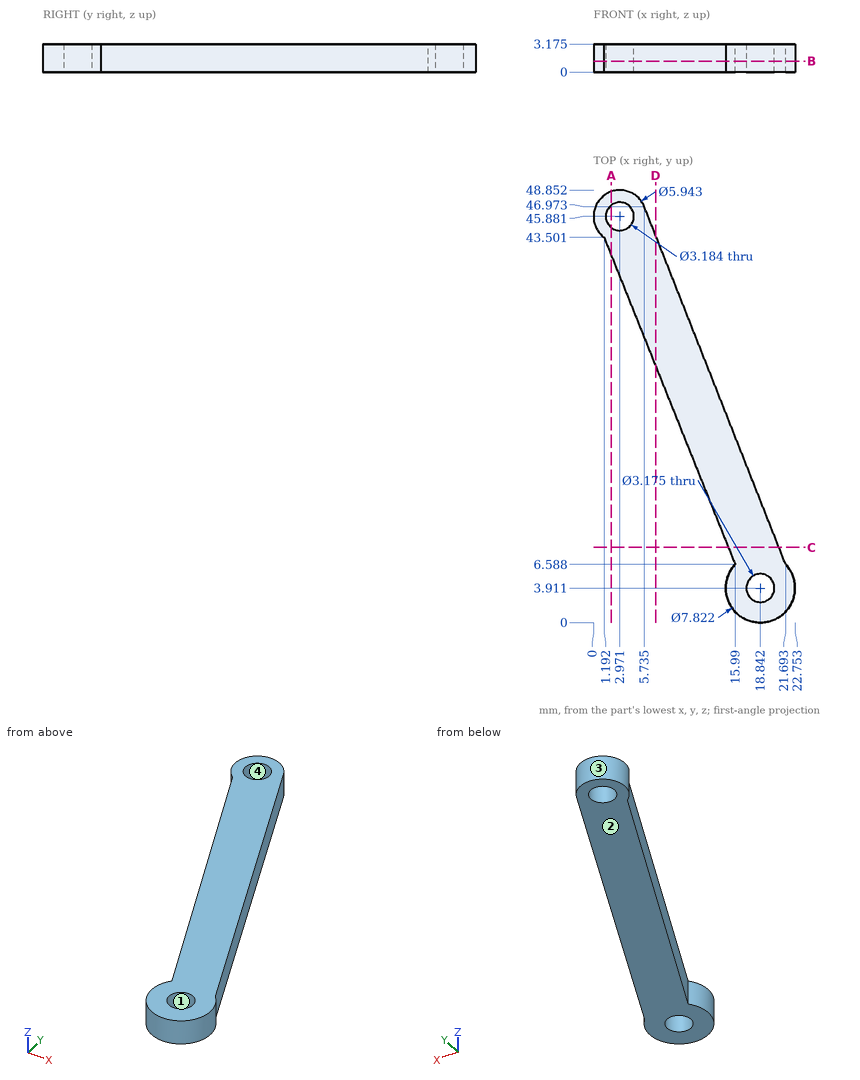
Print and shaded views of the part. All mm, measured from the part's lowest x, y and z. Coordinates: 2 decimals unless noted, no trailing zeros. Loops run counter-clockwise (first coordinate to the right, second up) from the corner with the lowest first, then second, coordinate; pieces in that order, holes last. Notation, with made-up numbers: (75.5, 61) - (121.5, 61) arc R22 ccw to (121.5, 88) - close; hole circle Ø6 at (85, 26). An arc over 180 degrees is marked (long way). Use one line per item in the form item = value. Start each with the question number.
1) Two-plate mould, pull along Y, no slides. Class the marked faces 1, 2, 3 and 4: +Y half, -Y half, draft (parallel to the pull), parting line (faces both ways), or undercut.
2) Band-saw the part on A-A (x = 2). Give the cut face in (y, z) (1 decimal).
3) Drill centre lines: L1, parallel to Y at x = 1.75, z = 2.7 (1 decimal); L2, parallel to X at y = 28.5, z = 0.15 (1 decimal); L3, parallel to X at y = 12.5, z = 3. Where is each one in solid material? Low to high. Write a range as from..to.
4) Band-saw the part on C-C (y = 8.5). Give the cut face in (x, z) (1 decimal).
5) Flat gauge pins, fed straight in: pin 1 (1 mm diameter, centred on x = 17, z = 2.5, fed in from -Y); pin 2 (2.5 mm diameter, centred on x = 2.97, y = 45.88, fed in from -Z). Where does each tip first touch, or does it go through?
6) Band-saw the part on D-D (x = 7). Give the cut face in (y, z) (1 decimal).
7) Band-saw the part on B-B (z = 1.25). Give the cut face in (x, y) (1 decimal), and give its area (3 significant figures).
Check values:
q1.face_1 = undercut
q1.face_2 = draft
q1.face_3 = parting line
q1.face_4 = undercut
q2.outline = (41.5, 0) - (44.6, 0) - (44.6, 3.2) - (41.5, 3.2) - close; (47.1, 0) - (48.7, 0) - (48.7, 3.2) - (47.1, 3.2) - close
q3.L1 = 42.1..44.9, 46.9..48.6
q3.L2 = 7.2..13
q3.L3 = 13.62..19.36
q4.outline = (15.2, 0) - (20.9, 0) - (20.9, 3.2) - (15.2, 3.2) - close
q5.pin_1 = 0.24
q5.pin_2 = through
q6.outline = (29, 0) - (43.8, 0) - (43.8, 3.2) - (29, 3.2) - close
q7.outline = (1.2, 43.5) - (16, 6.6) arc R3.9 ccw (long way) to (21.7, 6.6) - (5.7, 47) arc R3 ccw (long way) to start; hole circle Ø3.2 at (3, 45.9); hole circle Ø3.2 at (18.8, 3.9)
q7.area = 271 mm2
